Input: part model. Units: mm. Frame: model coordinates. A direction names the side the tool comes from. Coordinates: 2 decimals unless noted, no trailing zeros. Write each loop counter-clockwise with the first axis right and the second up, starting at its lowest first coordinate (ties: lowest second). Pieces come first, ordered by that corner, then holes.
1) Section query D-D (y = 717.5). Output: boundary loops of the cut face in (x, z).
2) Draft query along Z for faces 1 (the flat face through (533.4, 426, 126)), 2 (the flat face through (54, 101, 73.66)), 3 (the flat face through (13, 407.66, 141)). Return one class per face: pulls with the +Z half, pulls with the -Z half, needs draft (parallel to the pull), parting line crosses it, or undercut.
3) Set-up query: faces 4 (the flat face through (25.4, 645, 128)), 5 (the flat face through (279.4, 13, 141)), 6 (the flat face through (364.646, 444, 95)), 7 (the flat face through (13, 369, 205.74)). Return all of +Z, -Z, +X, -X, +Y, -Y with unobstructed straight access to the full face (end or side cutting, diameter ignored); none if empty.
4) Section query A-A (y = 445.5). Output: boundary loops of the cut face in (x, z), then the cut area to 3 significant figures.
5) Pin query (flat end, axial travel): pin 1 Ø8 at (x, y) = (214, 334.5) entering from +Z; pin 2 Ø8 at (x, y) = (158.5, 747) entering from -Z; pin 3 Ø5 at (x, z) = (402.5, 164.5) entering from +Y. Return the tip coordinate at first contact, or that it passes through.
6) Section query C-C (y = 108.5). Output: boundary loops of the cut face in (x, z), then the cut area to 3 significant figures.
7) Section query B-B (x = 116). Output: boundary loops of the cut face in (y, z).
8) Line query: L1, parallel to Y at x = 7.62, z = 246; L2, parallel to Y at x = 7, z = 250; L3, parallel to X at y = 855.98, z = 245.25. Output: solid intervals per line, ascending.
from build123d import *

# Parameters (mm, degrees)
F0_W      = 533.4
F0_H      = 863.6
F1_DEPTH  = 2.54
F2_W      = 533.4
F2_H      = 863.6
F2_W_2    = 482.6
F2_H_2    = 812.8
F3_DEPTH  = 254
F4_W      = 76.2
F4_H      = 330.2
F5_DEPTH  = 25.4
F6_W      = 177.8
F6_H      = 25.4
F6_W_2    = 279.4
F7_DEPTH  = 254
F8_W      = 25.4
F8_H      = 254
F8_H_2    = 127
F9_DEPTH  = 254
F10_W     = 76.2
F10_H     = 190.5
F10_H_2   = 187.96
F11_DEPTH = 25.4
F12_W     = 76.2
F12_H     = 190.5
F13_DEPTH = 25.4
F14_W     = 76.2
F14_H     = 190.5
F15_DEPTH = 25.4
F17_DEPTH = 25.4
F18_W     = 76.2
F18_H     = 127
F19_DEPTH = 25.4
F20_W     = 76.2
F20_H     = 127
F21_DEPTH = 25.4
F22_W     = 76.2
F22_H     = 127
F23_DEPTH = 25.4
F24_W     = 76.2
F24_H     = 127
F25_DEPTH = 25.4
F26_R     = 5.08
F27_DEPTH = 19.05
F28_R     = 5.08
F29_DEPTH = 25.4
F30_W     = 101.6
F30_H     = 203.2
F30_W_2   = 203.2
F30_H_2   = 152.4
F31_DEPTH = 63.5
F32_W     = 50.8
F32_H     = 25.4
F32_W_2   = 25.4
F32_H_2   = 50.8
F33_DEPTH = 7.62
F34_W     = 50.8
F34_H     = 101.6
F35_DEPTH = 152.4
F36_W     = 50.8
F36_H     = 25.4
F37_DEPTH = 50.8
F38_W     = 50.8
F38_H     = 25.4
F39_DEPTH = 25.4


with BuildPart() as f1:
    # F0 (on Top) → F1 (new body)
    with BuildSketch(Plane.XY):
        with Locations((266.7, 431.8)):
            Rectangle(F0_W, F0_H)
    extrude(amount=F1_DEPTH)

    # F2 (on face) → F3 (join)
    with BuildSketch(Plane.XY.offset(2.54)):
        with Locations((266.7, 431.8)):
            Rectangle(F2_W, F2_H)
        with Locations((266.7, 431.8)):
            Rectangle(F2_W_2, F2_H_2, mode=Mode.SUBTRACT)
    extrude(amount=F3_DEPTH)

    # F4 (on face) → F5 (cut)
    with BuildSketch(Plane.XY.offset(2.54)):
        with Locations((469.9, 190.5)):
            Rectangle(F4_W, F4_H)
    extrude(amount=-F5_DEPTH, mode=Mode.SUBTRACT)

    # F6 (on face) → F7 (join)
    with BuildSketch(Plane.XY.offset(2.54)):
        with Locations((419.1, 444.5)):
            Rectangle(F6_W, F6_H)
        Polygon((304.8, 431.8), (330.2, 431.8), (330.2, 457.2), (330.2, 838.2), (304.8, 838.2), (304.8, 457.2), align=None)
        with Locations((165.1, 444.5)):
            Rectangle(F6_W_2, F6_H)
    extrude(amount=F7_DEPTH)

    # F8 (on face) → F9 (join)
    with BuildSketch(Plane.XY.offset(2.54)):
        Polygon((152.4, 304.8), (25.4, 304.8), (25.4, 279.4), (406.4, 279.4), (431.8, 279.4), (431.8, 304.8), (177.8, 304.8), align=None)
        with Locations((419.1, 152.4)):
            Rectangle(F8_W, F8_H)
        with Locations((165.1, 368.3)):
            Rectangle(F8_W, F8_H_2)
    extrude(amount=F9_DEPTH)

    # F10 (on face) → F11 (cut)
    with BuildSketch(Plane.XZ.offset(-431.8)):
        with Locations((240.317534, 97.79)):
            Rectangle(F10_W, F10_H)
        with Locations((402.745839, 96.52)):
            Rectangle(F10_W, F10_H_2)
    extrude(amount=-F11_DEPTH, mode=Mode.SUBTRACT)

    # F12 (on face) → F13 (cut)
    with BuildSketch(Plane.YZ.offset(177.8)):
        with Locations((367.623325, 97.79)):
            Rectangle(F12_W, F12_H)
    extrude(amount=-F13_DEPTH, mode=Mode.SUBTRACT)

    # F14 (on face) → F15 (cut)
    with BuildSketch(Plane(origin=(0, 304.8, 0), x_dir=(-1, 0, 0), z_dir=(0, 1, 0))):
        with Locations((-314.105634, 97.79)):
            Rectangle(F14_W, F14_H)
    extrude(amount=-F15_DEPTH, mode=Mode.SUBTRACT)

    # F16 (on face) → F17 (cut)
    with BuildSketch(Plane.XZ.offset(-838.2)):
        Polygon((383.836448, 205.733197), (382.521942, 78.74), (460.036448, 78.74), (460.036448, 205.733197), align=None)
    extrude(amount=-F17_DEPTH, mode=Mode.SUBTRACT)

    # F18 (on face) → F19 (cut)
    with BuildSketch(Plane.XZ.offset(-838.2)):
        with Locations((165.1, 142.24)):
            Rectangle(F18_W, F18_H)
    extrude(amount=-F19_DEPTH, mode=Mode.SUBTRACT)

    # F20 (on face) → F21 (cut)
    with BuildSketch(Plane.YZ.offset(25.4)):
        with Locations((369.560152, 142.24)):
            Rectangle(F20_W, F20_H)
    extrude(amount=-F21_DEPTH, mode=Mode.SUBTRACT)

    # F22 (on face) → F23 (cut)
    with BuildSketch(Plane(origin=(0, 25.4, 0), x_dir=(-1, 0, 0), z_dir=(0, 1, 0))):
        with Locations((-317.5, 142.24)):
            Rectangle(F22_W, F22_H)
        with Locations((-114.3, 142.24)):
            Rectangle(F22_W, F22_H)
    extrude(amount=-F23_DEPTH, mode=Mode.SUBTRACT)

    # F24 (on face) → F25 (cut)
    with BuildSketch(Plane(origin=(508, 0, 0), x_dir=(0, -1, 0), z_dir=(-1, 0, 0))):
        with Locations((-369.560152, 142.24)):
            Rectangle(F24_W, F24_H)
    extrude(amount=-F25_DEPTH, mode=Mode.SUBTRACT)

    # F26 (on face) → F27 (join)
    with BuildSketch(Plane(origin=(0, 0, 0), x_dir=(1, 0, 0), z_dir=(0, 0, -1))):
        with Locations((7.62, -7.62)):
            Circle(F26_R)
        with Locations((525.78, -7.62)):
            Circle(F26_R)
        with Locations((525.78, -855.98)):
            Circle(F26_R)
        with Locations((7.62, -855.98)):
            Circle(F26_R)
    extrude(amount=F27_DEPTH)

    # F28 (on face) → F29 (cut)
    with BuildSketch(Plane.XY.offset(256.54)):
        with Locations((7.62, 7.62)):
            Circle(F28_R)
        with Locations((525.78, 7.62)):
            Circle(F28_R)
        with Locations((525.78, 855.98)):
            Circle(F28_R)
        with Locations((7.62, 855.98)):
            Circle(F28_R)
    extrude(amount=-F29_DEPTH, mode=Mode.SUBTRACT)

    # F30 (on face) → F31 (join)
    with BuildSketch(Plane.XY.offset(2.54)):
        with Locations((76.2, 736.6)):
            Rectangle(F30_W, F30_H)
        with Locations((457.2, 736.6)):
            Rectangle(F30_W, F30_H)
        with Locations((127, 144.306398)):
            Rectangle(F30_W_2, F30_H_2)
    extrude(amount=F31_DEPTH)

    # F32 (on face) → F33 (join)
    with BuildSketch(Plane.XY.offset(66.04)):
        with Locations((66.433271, 819.132545)):
            Rectangle(F32_W, F32_H)
        with Locations((455.950456, 819.132545)):
            Rectangle(F32_W, F32_H)
        with Locations((53.733271, 101.077922)):
            Rectangle(F32_W_2, F32_H_2)
        with Locations((53.733271, 184.012836)):
            Rectangle(F32_W_2, F32_H_2)
    extrude(amount=F33_DEPTH)

    # F34 (on face) → F35 (join)
    with BuildSketch(Plane.XY.offset(2.54)):
        with Locations((279.4, 746.542548)):
            Rectangle(F34_W, F34_H)
        with Locations((482.6, 508)):
            Rectangle(F34_W, F34_H)
        with Locations((381, 101.243105)):
            Rectangle(F34_W, F34_H)
    extrude(amount=F35_DEPTH)

    # F36 (on face) → F37 (join)
    with BuildSketch(Plane.XY.offset(2.54)):
        with Locations((60.292414, 317.5)):
            Rectangle(F36_W, F36_H)
        with BuildLine():
            add(Edge.make_bspline(
                [(60.37103, 381.865399), (27.375462, 381.865399), (43.873246, 343.765399), (60.37103, 305.665399), (76.868814, 343.765399), (93.366598, 381.865399), (60.37103, 381.865399)],
                knots=[0, 0, 0, 2.094395, 2.094395, 4.18879, 4.18879, 6.283185, 6.283185, 6.283185], degree=2, weights=[1, 0.5, 1, 0.5, 1, 0.5, 1]))
        make_face()
    extrude(amount=F37_DEPTH)

    # F38 (on face) → F39 (join)
    with BuildSketch(Plane.XY.offset(53.34)):
        with Locations((60.292414, 317.5)):
            Rectangle(F38_W, F38_H)
    extrude(amount=F39_DEPTH)


solid = f1.part
Answer:
1. outline: (0, 0) - (533.4, 0) - (533.4, 256.54) - (508, 256.54) - (508, 66.04) - (406.4, 66.04) - (406.4, 2.54) - (330.2, 2.54) - (330.2, 256.54) - (304.8, 256.54) - (304.8, 154.94) - (254, 154.94) - (254, 2.54) - (127, 2.54) - (127, 66.04) - (25.4, 66.04) - (25.4, 256.54) - (0, 256.54) - close
2. face 1: needs draft
2. face 2: pulls with the +Z half
2. face 3: undercut
3. face 4: +Z
3. face 5: -Y
3. face 6: none
3. face 7: -X
4. outline: (0, 0) - (533.4, 0) - (533.4, 256.54) - (0, 256.54) - close; hole (202.22, 2.54) - (278.42, 2.54) - (278.42, 193.04) - (202.22, 193.04) - close; hole (364.65, 2.54) - (440.85, 2.54) - (440.85, 190.5) - (364.65, 190.5) - close
4. area: 108,000 mm2
5. pin 1: stops at z = 2.54
5. pin 2: stops at z = 0
5. pin 3: stops at y = 304.8
6. outline: (0, 0) - (431.8, 0) - (431.8, 256.54) - (406.4, 256.54) - (406.4, 154.94) - (355.6, 154.94) - (355.6, 2.54) - (228.6, 2.54) - (228.6, 66.04) - (66.43, 66.04) - (66.43, 73.66) - (41.03, 73.66) - (41.03, 66.04) - (25.4, 66.04) - (25.4, 256.54) - (0, 256.54) - close; (508, 0) - (533.4, 0) - (533.4, 256.54) - (508, 256.54) - close
6. area: 41,400 mm2
7. outline: (0, 0) - (863.6, 0) - (863.6, 256.54) - (838.2, 256.54) - (838.2, 66.04) - (635, 66.04) - (635, 2.54) - (457.2, 2.54) - (457.2, 256.54) - (431.8, 256.54) - (431.8, 2.54) - (304.8, 2.54) - (304.8, 256.54) - (279.4, 256.54) - (279.4, 2.54) - (220.51, 2.54) - (220.51, 66.04) - (68.11, 66.04) - (68.11, 2.54) - (25.4, 2.54) - (25.4, 78.74) - (0, 78.74) - close; (0, 205.74) - (25.4, 205.74) - (25.4, 256.54) - (0, 256.54) - close
8. L1: y = 0 to 2.54, 12.7 to 850.9, 861.06 to 863.6
8. L2: y = 0 to 2.58, 12.66 to 850.94, 861.02 to 863.6
8. L3: x = 0 to 2.54, 12.7 to 520.7, 530.86 to 533.4
